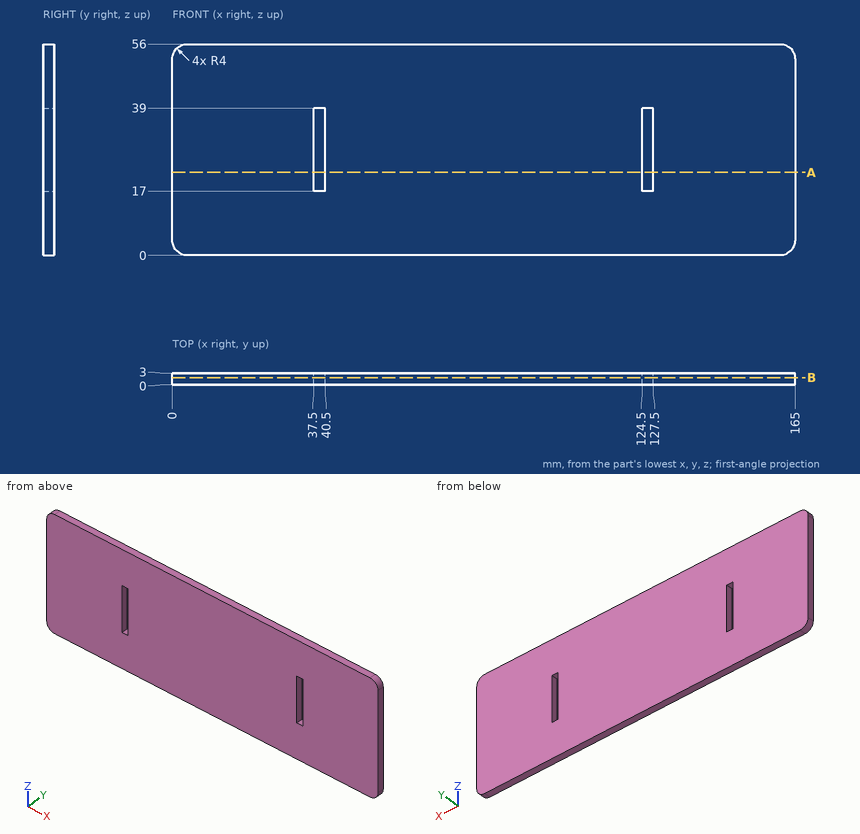
For this review, use the dimensioned drawing (mm, ordinates from the lowest corner) and the shaded views. Coordinates: 2 decimals unless noted, no trailing zeros. Order: outer loops, then holes, each group sorted by start corner. A loop starts at its lowest first (then second) coordinate and runs counter-clockwise, first axis right, second up. Notation, with made-up numbers: (71, 64) - (108, 64) arc R10 ccw to (108, 70) - close; hole circle Ø7 at (4.25, -2). An arc over 180 degrees is marked (long way). Answer as a JSON object with one key per item and string values. Group by question number.
1. We need section B-B on y = 1.85. State the section outline as (x, z) points, then the cut area to 3 significant figures.
2. We need section A-A on z = 22. State the section outline as (x, y) points.
3. For probe 1 along X at (y, z) = (2, 36); probe 2 along Z at (x, y) = (38, 1.8), list the stretches that pass through material, from the lowest coordinate up.
Final values:
{
 "1": {"outline": "(0, 4) arc R4 ccw to (4, 0) - (161, 0) arc R4 ccw to (165, 4) - (165, 52) arc R4 ccw to (161, 56) - (4, 56) arc R4 ccw to (0, 52) - close; hole (37.5, 17) - (40.5, 17) - (40.5, 39) - (37.5, 39) - close; hole (124.5, 17) - (127.5, 17) - (127.5, 39) - (124.5, 39) - close", "area": "9,090 mm²"},
 "2": {"outline": "(0, 0) - (37.5, 0) - (37.5, 3) - (0, 3) - close; (40.5, 0) - (124.5, 0) - (124.5, 3) - (40.5, 3) - close; (127.5, 0) - (165, 0) - (165, 3) - (127.5, 3) - close"},
 "3": {"probe 1": "0 to 37.5, 40.5 to 124.5, 127.5 to 165", "probe 2": "0 to 17, 39 to 56"}
}
